Read the model definition and answer for the solid it produces. Units are mm, in the model's axes. Face numbers are marked on the shaded views. Round coordinates to 2 decimals unless told otherwise and drop trailing zeros. Write each loop counter-clockwise with the first axis right and the second up, starting at its lowest first coordinate (ties: lowest second). Pieces come first, ordered by that corner, then holes.
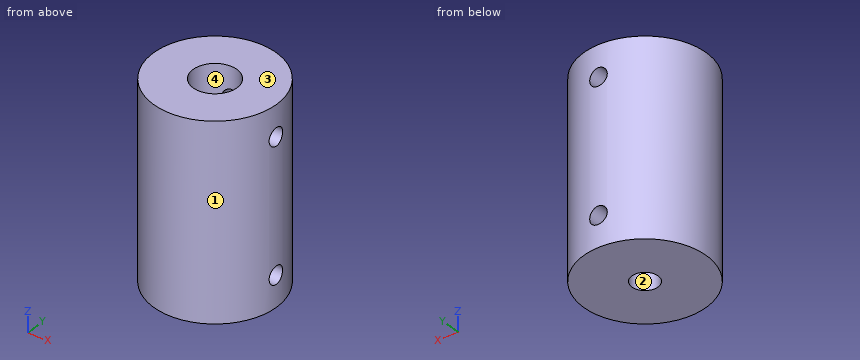
Autodesk Fusion 360 part; units mm, degrees
sketch "スケッチ1" plane through (0, 0, 0) normal (0, 0, 1) x (1, 0, 0)
  circle A0 centre (0, 0) radius 7
  dimension "d1" = 14
extrude "押し出し1" add sketch "スケッチ1" along normal blind 12
extrude "押し出し2" add 1 faces at (1.11, -1.8763, 12) along direction (0, 0, 1) blind 10
sketch "スケッチ2" plane through (0, 0, 22) normal (0, 0, 1) x (-1, 0, 0)
  circle A0 centre (0, 0) radius 7
  circle A1 centre (0, 0) radius 2.5
  dimension "d6" = 5
sketch "スケッチ3" plane through (0, 0, 0) normal (0, 0, -1) x (1, 0, 0)
  circle A0 centre (0, 0) radius 7
  circle A1 centre (0, 0) radius 1.5
  dimension "d7" = 3
extrude "押し出し3" cut sketch "スケッチ3" against normal blind 11 contours A1
extrude "押し出し4" cut sketch "スケッチ2" against normal blind 11 contours A1
sketch "スケッチ4" plane through (0, 0, 0) normal (0, 1, 0) x (1, 0, 0)
  line L0 (-7, -22) -> (7, -22)
  line L1 (7, -22) -> (7, 0)
  line L2 (7, 0) -> (-7, 0)
  line L3 (-7, 0) -> (-7, -22)
  line L4 (-7, -22) -> (-7, -18.5)
  line L5 (-7, -18.5) -> (7, -18.5)
  line L6 (7, -22) -> (7, -18.5)
  line L7 (0, -22) -> (0, 0)
  circle A0 centre (0, -18.5) radius 1
  line L8 (-7, 0) -> (-7, -3.5)
  line L9 (-7, -3.5) -> (7, -3.5)
  circle A1 centre (0, -3.5) radius 1
  dimension "d12" = 3.5
  dimension "d13" = 2
  dimension "d20" = 3.5
  dimension "d21" = 2
extrude "押し出し5" cut sketch "スケッチ4" along normal blind 10 contours L5 L7 A0 | L5 L7 A0 | L5 L7 A0 | L5 L7 A0
sketch "スケッチ5" plane through (0, 0, 0) normal (1, 0, 0) x (0, 1, 0)
  line L0 (-7, 22) -> (7, 22)
  line L1 (7, 22) -> (7, 0)
  line L2 (7, 0) -> (-7, 0)
  line L3 (-7, 0) -> (-7, 22)
  line L4 (-7, 22) -> (-7, 18.5)
  line L5 (-7, 22) -> (7, 22)
  line L6 (7, 22) -> (7, 18.5)
  line L7 (7, 18.5) -> (-7, 18.5)
  line L8 (-7, 18.5) -> (-7, 22)
  circle A0 centre (0, 18.5) radius 1
  line L9 (7, 0) -> (7, 3.5)
  line L10 (7, 3.5) -> (-7, 3.5)
  circle A1 centre (0, 3.5) radius 1
  dimension "d16" = 3.5
  dimension "d17" = 2
  dimension "d24" = 3.5
  dimension "d25" = 2
extrude "押し出し6" cut sketch "スケッチ5" along normal blind 10 contours L7 A0 | L7 A0
extrude "押し出し7" cut sketch "スケッチ4" along normal blind 10 contours L7 L9 A1 | L7 L9 A1 | L7 L9 A1 | L7 L9 A1
extrude "押し出し8" cut sketch "スケッチ5" along normal blind 10 contours L10 A1 | L10 A1
Q1. Section C-C (z = 9.75) is taken. Determine the outline of the cut face in (x, y).
Verdict:
outline: circle Ø14 at (0, 0); hole circle Ø3 at (0, 0)
Q2. Section A-A (x = 0) is taken. Determine the outline of the cut face in (y, z).
Verdict:
outline: (-7, 0) - (-1.5, 0) - (-1.5, 11) - (-2.5, 11) - (-2.5, 22) - (-7, 22) - close; (1.5, 0) - (7, 0) - (7, 2.5) - (1.5, 2.5) - close; (1.5, 4.5) - (7, 4.5) - (7, 17.5) - (2.5, 17.5) - (2.5, 11) - (1.5, 11) - close; (2.5, 19.5) - (7, 19.5) - (7, 22) - (2.5, 22) - close
Q3. Determine the mould class of the marked faces 1, 2, 3 and 4 for opening direction X: pulls with the +X half, pulls with the -X half, needs draft (parallel to the pull), parting line crosses it, or undercut.
Verdict:
face 1: parting line crosses it
face 2: undercut
face 3: needs draft
face 4: undercut
Q4. Straight lines are drawn through the part: probe 1 along Y at (x, z) = (0, 15.25); probe 2 along Z at (x, y) = (5.15, 0); probe 3 along X at (y, z) = (-1, 14). For each, find the intervals that lie inside material, in ascending order.
Verdict:
probe 1: y = -7 to -2.5, 2.5 to 7
probe 2: z = 0 to 2.5, 4.5 to 17.5, 19.5 to 22
probe 3: x = -6.93 to -2.29, 2.29 to 6.93
Q5. Flat-ended cylindrical pins translate along their axes: pin 1 Ø1.2 at (x, z) = (0, 18.5) entering from +Y; pin 2 Ø1.6 at (y, z) = (0, 3.5) entering from +X; pin 3 Ø1 at (x, z) = (3.5, 15.5) entering from -Y; pin 4 Ø2.5 at (x, y) = (0, 0) entering from -Z. Find the tip coordinate at first contact, or state that the pin passes through.
Verdict:
pin 1: stops at y = -2.43
pin 2: stops at x = -1.27
pin 3: stops at y = -6.32
pin 4: passes through
Q6. Section D-D (y = 6) is taken. Determine the outline of the cut face in (x, z), then the cut area to 3 significant figures.
Verdict:
outline: (-3.61, 0) - (3.61, 0) - (3.61, 22) - (-3.61, 22) - close; hole circle Ø2 at (0, 3.5); hole circle Ø2 at (0, 18.5)
area: 152 mm2
